Check sheet for the modelled part. Datum: model origin and axes. Units: mm. Give positions to 0.01 mm unless a question says otherwise; leave off trailing zeros. Loops run counter-clockwise (first coordinate to the right, second up) from the corner with the lowest first, then second, coordinate; pieces in that order, holes last. Notation, with made-up numbers: (52.25, 50) - (80.25, 50) arc R29 ccw to (80.25, 77) - close; hole circle Ø11 at (21.5, -10.75). An arc over 180 degrees is marked (long way). Answer in a Markdown table with one row per item. Add a question column.
(1) Sectioned sample at B-B on x = 129.5. Enter the section's corners in (y, z), then the cut area to 3 significant figures.
(2) Sectioned sample at C-C on z = 3.4. State how many separate pieces and enclosed holes the cut face has, then the cut area to 3 significant figures.
(3) Sectioned sample at A-A on y = 112. Enter the section's corners in (x, z), then the cut area to 3 significant figures.
(4) Go/stop test with flat-tipped pins: P1, Ø1.5, axis at x = 78.5, z = 3, coming from the -Y side; P2, Ø1.6, axis at y = 49.5, z = 2, coming from the -X side. Record where each tip stops, or that it passes through.
(5) Thickness scan on L1, parallel to X at y = 105.5, z = 2.25; L2, parallel to Y at x = 78.5, z = 2; L3, parallel to Y at x = 132, z = 0.35. Record the ranges inside material, lowest first.
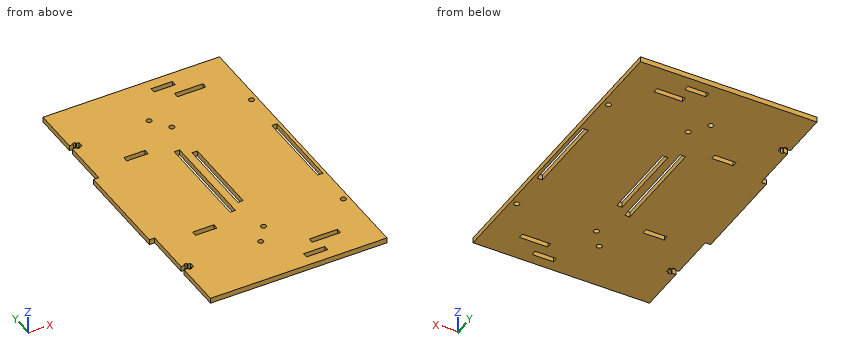
from build123d import *

# Parameters (mm, degrees)
CROQUIS1_W              = 5
CROQUIS1_H              = 93.333333334
SALIENTE_EXTRUIR1_DEPTH = 5
CORTAR_EXTRUIR1_DEPTH   = 5
CROQUIS3_W              = 5
CROQUIS3_H              = 93.333333334
CORTAR_EXTRUIR2_DEPTH   = 5
CROQUIS4_R              = 2.5
CORTAR_EXTRUIR3_DEPTH   = 5
CROQUIS5_W              = 20
CROQUIS5_H              = 5
CORTAR_EXTRUIR4_DEPTH   = 5
CROQUIS6_W              = 40
CROQUIS6_H              = 280
SALIENTE_EXTRUIR2_DEPTH = 5
CROQUIS7_W              = 5
CROQUIS7_H              = 76.666666666
CROQUIS7_W_2            = 26.666666666
CROQUIS7_H_2            = 5
CROQUIS7_R              = 2.5
CORTAR_EXTRUIR5_DEPTH   = 5


with BuildPart() as part:
    # Croquis1 → Saliente-Extruir1 (new body)
    with BuildSketch(Plane.XY):
        Polygon((5, 93.333333333), (5, 0), (131, 0), (131, 93.333333333), (131, 186.666666667), (131, 280), (5, 280), (5, 186.666666667), align=None)
        with Locations((2.5, 140)):
            Rectangle(CROQUIS1_W, CROQUIS1_H)
    extrude(amount=SALIENTE_EXTRUIR1_DEPTH)

    # Croquis2 → Cortar-Extruir1 (cut)
    with BuildSketch(Plane.XY.offset(5)):
        Polygon((8.7, 235.833333333), (5, 235.833333333), (5, 230.833333333), (8.7, 230.833333333), (8.7, 229.333333333), (11.5, 229.333333333), (11.5, 230.833333333), (14, 230.833333333), (14, 235.833333333), (11.5, 235.833333333), (11.5, 237.333333333), (8.7, 237.333333333), align=None)
        Polygon((8.7, 49.166666667), (5, 49.166666667), (5, 44.166666667), (8.7, 44.166666667), (8.7, 42.666666667), (11.5, 42.666666667), (11.5, 44.166666667), (14, 44.166666667), (14, 49.166666667), (11.5, 49.166666667), (11.5, 50.666666667), (8.7, 50.666666667), align=None)
    extrude(amount=-CORTAR_EXTRUIR1_DEPTH, mode=Mode.SUBTRACT)

    # Croquis3 → Cortar-Extruir2 (cut)
    with BuildSketch(Plane.XY.offset(5)):
        with Locations((78.5, 140)):
            Rectangle(CROQUIS3_W, CROQUIS3_H)
    extrude(amount=-CORTAR_EXTRUIR2_DEPTH, mode=Mode.SUBTRACT)

    # Croquis4 → Cortar-Extruir3 (cut)
    with BuildSketch(Plane.XY.offset(5)):
        with Locations((78.5, 233.333333333)):
            Circle(CROQUIS4_R)
        with Locations((78.5, 46.666666667)):
            Circle(CROQUIS4_R)
    extrude(amount=-CORTAR_EXTRUIR3_DEPTH, mode=Mode.SUBTRACT)

    # Croquis5 → Cortar-Extruir4 (cut)
    with BuildSketch(Plane.XY.offset(5)):
        with Locations((46, 197.5)):
            Rectangle(CROQUIS5_W, CROQUIS5_H)
        with Locations((111, 267.5)):
            Rectangle(CROQUIS5_W, CROQUIS5_H)
        with Locations((46, 82.5)):
            Rectangle(CROQUIS5_W, CROQUIS5_H)
        with Locations((111, 12.5)):
            Rectangle(CROQUIS5_W, CROQUIS5_H)
    extrude(amount=-CORTAR_EXTRUIR4_DEPTH, mode=Mode.SUBTRACT)

    # Croquis6 → Saliente-Extruir2 (add)
    with BuildSketch(Plane.XY.offset(5)):
        with Locations((151, 140)):
            Rectangle(CROQUIS6_W, CROQUIS6_H)
    extrude(amount=-SALIENTE_EXTRUIR2_DEPTH)

    # Croquis7 → Cortar-Extruir5 (cut)
    with BuildSketch(Plane.XY.offset(5)):
        with Locations((90.5, 140)):
            Rectangle(CROQUIS7_W, CROQUIS7_H)
        with Locations((165.5, 140)):
            Rectangle(CROQUIS7_W, CROQUIS7_H)
        with Locations((128, 27.5)):
            Rectangle(CROQUIS7_W_2, CROQUIS7_H_2)
        with Locations((128, 252.5)):
            Rectangle(CROQUIS7_W_2, CROQUIS7_H_2)
        with Locations((90.5, 216.666666667)):
            Circle(CROQUIS7_R)
        with Locations((165.5, 216.666666667)):
            Circle(CROQUIS7_R)
        with Locations((165.5, 63.333333333)):
            Circle(CROQUIS7_R)
        with Locations((90.5, 63.333333333)):
            Circle(CROQUIS7_R)
    extrude(amount=-CORTAR_EXTRUIR5_DEPTH, mode=Mode.SUBTRACT)


solid = part.part
Reply:
| question | item | result |
|---|---|---|
| 1 | outline | (0, 0) - (25, 0) - (25, 5) - (0, 5) - close; (30, 0) - (250, 0) - (250, 5) - (30, 5) - close; (255, 0) - (280, 0) - (280, 5) - (255, 5) - close |
| 1 | area | 1,350 mm^2 |
| 2 | separate pieces | 1 |
| 2 | enclosed holes | 15 |
| 2 | area | 44,800 mm^2 |
| 3 | outline | (0, 0) - (76, 0) - (76, 5) - (0, 5) - close; (81, 0) - (88, 0) - (88, 5) - (81, 5) - close; (93, 0) - (163, 0) - (163, 5) - (93, 5) - close; (168, 0) - (171, 0) - (171, 5) - (168, 5) - close |
| 3 | area | 780 mm^2 |
| 4 | P1 | y = 0 |
| 4 | P2 | x = 5 |
| 5 | L1 | 0 to 76, 81 to 88, 93 to 163, 168 to 171 |
| 5 | L2 | 0 to 44.17, 49.17 to 93.33, 186.67 to 230.83, 235.83 to 280 |
| 5 | L3 | 0 to 25, 30 to 250, 255 to 280 |
